Work out the finished part from the listing and answer in its coordinate system (mm). A direction names the side the tool comes from. Give positions to 0.01 mm unless a question says otherwise; leave off trailing zeros. Order: outer loops, then holes, each group sorted by start corner. A loop starts at its lowest first (then second) coordinate and runs counter-clockwise, first axis right, second up. Notation, with made-up numbers: (-17.5, 27) - (22.5, 27) arc R23 cw to (22.5, 35) - close; hole circle Ø1 at (-24, 77). An arc over 180 degrees is marked (long way). Return JSON: item names as keys, results as strings. Group by question number.
from build123d import *

# Parameters (mm, degrees)
SKETCH1_R           = 3.1
SKETCH1_R_2         = 2.4
BOSS_EXTRUDE1_DEPTH = 1.7
SKETCH2_R           = 3.95
BOSS_EXTRUDE2_DEPTH = 1
SKETCH3_R           = 2.4
BOSS_EXTRUDE3_DEPTH = 1.7


with BuildPart() as part:
    # Sketch1 → Boss-Extrude1 (new body)
    with BuildSketch(Plane(origin=(0, 0, 0), x_dir=(1, 0, 0), z_dir=(0, 1, 0))):
        with Locations(Location((0, 0, 0), (0, 0, 270))):
            Circle(SKETCH1_R)
        with Locations(Location((0, 0, 0), (0, 0, 270))):
            Circle(SKETCH1_R_2, mode=Mode.SUBTRACT)
    extrude(amount=BOSS_EXTRUDE1_DEPTH)

    # Sketch2 → Boss-Extrude2 (add)
    with BuildSketch(Plane(origin=(0, 1.7, 0), x_dir=(1, 0, 0), z_dir=(0, 1, 0))):
        with Locations(Location((0, 0, 0), (0, 0, 270))):
            Circle(SKETCH2_R)
    extrude(amount=BOSS_EXTRUDE2_DEPTH)

    # Sketch3 → Boss-Extrude3 (add)
    with BuildSketch(Plane(origin=(0, 2.7, 0), x_dir=(1, 0, 0), z_dir=(0, 1, 0))):
        with Locations(Location((0, 0, 0), (0, 0, 270))):
            Circle(SKETCH3_R)
    extrude(amount=BOSS_EXTRUDE3_DEPTH)


solid = part.part
1. Determine the mould class of faces 1 (the cylindrical face through (2.024, 0.838, 1.29)), 2 (the flat face through (-2, 2.7, 2)), 3 (the flat face through (0, 1.7, 0)), 4 (the cylindrical face through (2.67, 2.19, -2.91)) for opening direction X: released by +X, released by -X, zero draft, split by the parting line, or undercut.
2. The part is cut by section D-D (y = 3.3). Give the vertices of the cut face in (x, z).
3. The part is cut by section A-A (z = 0). Give the vertices of the cut face in (x, y), and give its area (3 significant figures).
4. Consider probe 1 along X at (y, z) = (0.4, 0); probe 2 along Y at (x, z) = (0, 0.5); probe 3 along Y at (x, z) = (-3.5, -0.5). Determine where each line is inside the solid, lowest interval first. Write a range as from..to.
5. Each of these flat-tipped pins is pushed along its axis until it touches: pin 1 (4 mm diameter, centred on x = -2.5, z = 0.5, fed in from +Y); pin 2 (4 mm diameter, centred on x = 0, z = 0, fed in from -Y). Where does it stop, or does it pass through?
6. A tool of negligible diameter and unlimited length cuts with its end or side. For faces 5 (the cylindrical face through (0.931, 0.838, 2.957)), 6 (the cylindrical face through (2.024, 3.538, 1.29)), 7 (the flat face through (0, 4.4, 0)), from which of +Z, -Z, +X, -X, +Y, -Y can it reach the whole face along a straight path? Write none if from no direction.
7. The part is cut by section B-B (x = 0). Give the vertices of the cut face in (y, z).
8. The part is cut by section C-C (y = 0.35). Give the vertices of the cut face in (x, z), and give its area (3 significant figures).
Answers:
{
 "1": {"face 1": "undercut", "face 2": "zero draft", "face 3": "undercut", "face 4": "split by the parting line"},
 "2": {"outline": "circle Ø4.8 at (0, 0)"},
 "3": {"outline": "(-3.95, 1.7) - (-3.1, 1.7) - (-3.1, 0) - (-2.4, 0) - (-2.4, 1.7) - (2.4, 1.7) - (2.4, 0) - (3.1, 0) - (3.1, 1.7) - (3.95, 1.7) - (3.95, 2.7) - (2.4, 2.7) - (2.4, 4.4) - (-2.4, 4.4) - (-2.4, 2.7) - (-3.95, 2.7) - close", "area": "18.4 mm^2"},
 "4": {"probe 1": "x = -3.1..-2.4, 2.4..3.1", "probe 2": "y = 1.7..4.4", "probe 3": "y = 1.7..2.7"},
 "5": {"pin 1": "stops at y = 4.4", "pin 2": "stops at y = 1.7"},
 "6": {"face 5": "-Y", "face 6": "+Y", "face 7": "+Z, -Z, +X, -X, +Y"},
 "7": {"outline": "(0, -3.1) - (1.7, -3.1) - (1.7, -3.95) - (2.7, -3.95) - (2.7, -2.4) - (4.4, -2.4) - (4.4, 2.4) - (2.7, 2.4) - (2.7, 3.95) - (1.7, 3.95) - (1.7, 3.1) - (0, 3.1) - (0, 2.4) - (1.7, 2.4) - (1.7, -2.4) - (0, -2.4) - close"},
 "8": {"outline": "circle Ø6.2 at (0, 0); hole circle Ø4.8 at (0, 0)", "area": "12.1 mm^2"}
}
